```python
from build123d import *

# Parameters (mm, degrees)
F0_W         = 16
F0_H         = 7.6
F1_DEPTH     = 3
F2_R         = 1.1
F3_DEPTH     = 1.7
F5_R         = 1.2
F6_DEPTH     = 3
F6_TAPER     = 7
F7_S5_R      = 1.1
F7_T6_DEPTH  = 3
F7_S11_R     = 1.1
F7_T12_DEPTH = 3
F4_W         = 16
F4_H         = 6
F8_DEPTH     = 7.7
F9_R         = 3
F10_DEPTH    = 5
F11_W        = 1.2
F11_H        = 3.5
F12_DEPTH    = 7.7
F13_R        = 1.5
F14_R        = 0.5
F16_DEPTH    = 4.7
F17_DEPTH    = 7.7
F18_SIZE     = 3
F19_R        = 1


# Not quite as in the source:
# - a fillet or chamfer that OpenCascade refuses, or shapes differently, is made with other operations: its cross-section is extruded or revolved along the edge and cut away or added


with BuildPart() as f1:
    # F0 (on Top) → F1 (new body)
    with BuildSketch(Plane.XY):
        Rectangle(F0_W, F0_H)
    extrude(amount=F1_DEPTH)

    # F2 (on face) → F3 (join)
    with BuildSketch(Plane.XY.offset(3)):
        with Locations((-4.75, 0)):
            Circle(F2_R)
        with Locations((4.75, 0)):
            Circle(F2_R)
    extrude(amount=F3_DEPTH)

    # F5 (on face) → F6 (join)
    with BuildSketch(Plane.XY.offset(4.7)):
        with Locations((-4.75, 0)):
            Circle(F5_R)
        with Locations((4.75, 0)):
            Circle(F5_R)
    extrude(amount=F6_DEPTH, taper=F6_TAPER)

    # F7: fillet of radius 0.1 on 2 edges, made by hand


with BuildPart() as f7_tool2:
    # F7_s3 → F7_t4 (revolve)
    with BuildSketch(Plane.XZ):
        with BuildLine():
            ThreePointArc((-3.6630294386, 4.7), (-3.5881338666, 4.7337379952), (-3.5637748235, 4.8121869343))
            Line((-3.5637748235, 4.8121869343), (-3.55, 4.7))
            Line((-3.55, 4.7), (-3.6630294386, 4.7))
        make_face()
    revolve(axis=Axis((-4.75, 0, 4.7), (0, 0, -1)))

    # F7_s5 → F7_t6 (cut, symmetric)
    with BuildSketch(Plane.XY.offset(4.8)):
        with Locations((-4.75, 0)):
            Circle(F7_S5_R)
    extrude(amount=F7_T6_DEPTH, both=True, mode=Mode.SUBTRACT)


with BuildPart() as f1_1:
    add(f1.part)

    # F7_t1: cut F7_tool2
    add(f7_tool2.part, mode=Mode.SUBTRACT)


with BuildPart() as f7_tool8:
    # F7_s9 → F7_t10 (revolve)
    with BuildSketch(Plane.XZ):
        with BuildLine():
            ThreePointArc((5.8369705614, 4.7), (5.9118661334, 4.7337379952), (5.9362251765, 4.8121869343))
            Line((5.9362251765, 4.8121869343), (5.95, 4.7))
            Line((5.95, 4.7), (5.8369705614, 4.7))
        make_face()
    revolve(axis=Axis((4.75, 0, 4.7), (0, 0, -1)))

    # F7_s11 → F7_t12 (cut, symmetric)
    with BuildSketch(Plane.XY.offset(4.8)):
        with Locations((4.75, 0)):
            Circle(F7_S11_R)
    extrude(amount=F7_T12_DEPTH, both=True, mode=Mode.SUBTRACT)


with BuildPart() as f1_2:
    add(f1_1.part)

    # F7_t7: cut F7_tool8
    add(f7_tool8.part, mode=Mode.SUBTRACT)

    # F4 (on Top) → F8 (join, through all)
    with BuildSketch(Plane.XY):
        with Locations((0, 6.8)):
            Rectangle(F4_W, F4_H)
    extrude(amount=F8_DEPTH)

    # F9 (on face) → F10 (join)
    with BuildSketch(Plane(origin=(0, 9.8, 0), x_dir=(-1, 0, 0), z_dir=(0, 1, 0))):
        with BuildLine():
            ThreePointArc((1.6785410332, 0), (3.5135361347, 1.5488994306), (4.2, 3.85))
            ThreePointArc((4.2, 3.85), (3.5135361347, 6.1511005694), (1.6785410332, 7.7))
            Line((1.6785410332, 7.7), (-1.6785410332, 7.7))
            ThreePointArc((-1.6785410332, 7.7), (-4.2, 3.85), (-1.6785410332, 0))
            Line((-1.6785410332, 0), (1.6785410332, 0))
        make_face()
        with Locations((0, 3.85)):
            Circle(F9_R, mode=Mode.SUBTRACT)
    extrude(amount=F10_DEPTH)

    # F11 (on face) → F12 (cut, through all)
    with BuildSketch(Plane.XY.offset(7.7)):
        with Locations((0, 13.05)):
            Rectangle(F11_W, F11_H)
    extrude(amount=-F12_DEPTH, mode=Mode.SUBTRACT)

    # F13
    f13_edges = [f1_2.edges().sort_by_distance(p)[0] for p in [
        (-8, -3.8, 1.5),
        (8, -3.8, 1.5),
    ]]
    fillet(f13_edges, radius=F13_R)

    # F14
    f14_edges = [f1_2.edges().sort_by_distance(p)[0] for p in [
        (-0.6, 11.3, 7.244694),
        (0.6, 11.3, 7.244694),
        (0.6, 11.3, 0.455306),
        (-0.6, 11.3, 0.455306),
    ]]
    fillet(f14_edges, radius=F14_R)

    # F15 (on face) → F16 (cut, through all)
    with BuildSketch(Plane.XY.offset(7.7)):
        with BuildLine():
            ThreePointArc((3.0310889132, 3.8), (3.380740392, 4.6441333421), (3.5, 5.55))
            ThreePointArc((3.5, 5.55), (-0.9058666579, 8.930740392), (-3.0310889132, 3.8))
            Line((-3.0310889132, 3.8), (0, 3.8))
            Line((0, 3.8), (3.0310889132, 3.8))
        make_face()
        with BuildLine():
            ThreePointArc((1.75, 5.55), (1.2374368671, 4.3125631329), (0, 3.8))
            ThreePointArc((0, 3.8), (-1.2374368671, 6.7874368671), (1.75, 5.55))
        make_face(mode=Mode.SUBTRACT)
        with BuildLine():
            ThreePointArc((1.75, 5.55), (-1.2374368671, 6.7874368671), (0, 3.8))
            ThreePointArc((0, 3.8), (1.2374368671, 4.3125631329), (1.75, 5.55))
        make_face()
    extrude(amount=-F16_DEPTH, mode=Mode.SUBTRACT)

    # F15 (on face) → F17 (cut, through all)
    with BuildSketch(Plane.XY.offset(7.7)):
        with BuildLine():
            ThreePointArc((1.75, 5.55), (-1.2374368671, 6.7874368671), (0, 3.8))
            ThreePointArc((0, 3.8), (1.2374368671, 4.3125631329), (1.75, 5.55))
        make_face()
    extrude(amount=-F17_DEPTH, mode=Mode.SUBTRACT)

    # F18
    f18_edges = [f1_2.edges().sort_by_distance(p)[0] for p in [
        (-8, 9.8, 3.85),
        (8, 9.8, 3.85),
    ]]
    chamfer(f18_edges, length=F18_SIZE)

    # F19
    f19_edges = [f1_2.edges().sort_by_distance(p)[0] for p in [
        (-4.2, 9.8, 3.85),
        (4.2, 9.8, 3.85),
    ]]
    fillet(f19_edges, radius=F19_R)


solid = f1_2.part
```
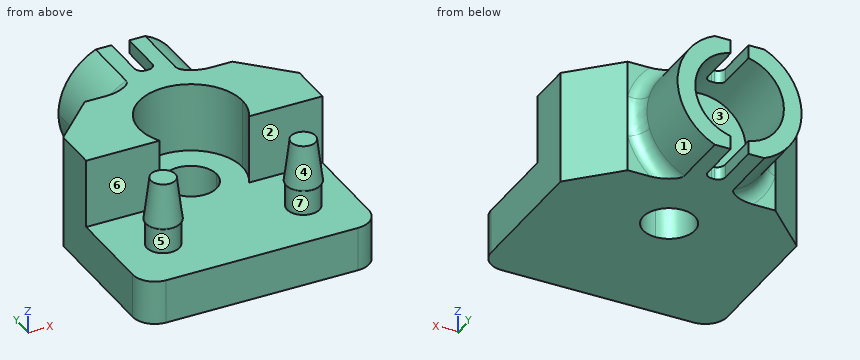
Input: part model. Units: mm. Frame: model coordinates. Face numbers are marked on the shaded views. A direction names the side the tool comes from. Give positions to 0.01 mm unless a question says otherwise; leave off trailing zeros. Order: outer loops, then holes, each group sorted by start corner. A loop starts at its lowest first (then second) coordinate and runs counter-clockwise, first axis right, second up. Notation, with made-up numbers: M -1.5,-5.5 L 6.5,-5.5 A4 cw 6.5,-0.5 Z; hole C 81,87.5 d11. An arc over 180 degrees is marked long. One line per question, with ' | ' between items. Start each with the question number.
1. Section query B-B (z = 6.5). Count the separate pieces of the cut face and the enclosed holes in it, and give its area (3 significant figures).
2. Access query for the marked faces 1, 2 and 3. Directions: +Z, -Z, +X, -X, +Y, -Y. A direction counts if a zero-diameter tool reaches every point of the face in a straight line with its end or side. Return the directions, or none.
3. Pull-direction query (Z, two-part tool) for the marked faces 4, 5, 6 and 7; classes: released by +Z, released by -Z, zero draft, split by the parting line, or undercut.
4. Material intervals for probe 1 along X at (y, z) = (5.55, 4); probe 2 along X at (y, z) = (5.55, 1.1); probe 3 along Y at (x, z) = (0, 5.65), sorted ascending. Write a range as [from, to].
5. First-contact query: pin 1 Ø3 at (x, y) = (0, 5.55) entering from -Z; pin 2 Ø1 at (y, z) = (14, 7) entering from -X; pin 3 Ø1.8 at (x, z) = (-0.5, 2.5) entering from +Y; pin 4 Ø4 at (x, y) = (0.5, 5) entering from +Z. Flat tips, straight axial feed; report the tip coordinate or a pass-through.
6. Section query C-C (y = 8.25). Return the cut outline in (x, z).
7. Section query A-A (y = 0). Return the cut outline in (x, z).
Here are the results:
1) separate pieces: 3 | enclosed holes: 0 | area: 81.1 mm²
2) face 1: +X, +Y | face 2: +Z, +X, -X | face 3: +Y
3) face 4: released by +Z | face 5: undercut | face 6: zero draft | face 7: undercut
4) probe 1: [-8, -3.5], [3.5, 8] | probe 2: [-8, -1.75], [1.75, 8] | probe 3: [9.05, 9.8]
5) pin 1: through | pin 2: x = -3.26 | pin 3: y = 9.8 | pin 4: z = 3
6) outline: M -6.55,0 L 6.55,0 L 6.55,7.7 L 2.23,7.7 L 2.23,3 L -2.23,3 L -2.23,7.7 L -6.55,7.7 Z
7) outline: M -8,0 L 8,0 L 8,3 L 5.85,3 L 5.85,4.7 A0.1 ccw 5.94,4.81 L 5.58,7.7 L 3.92,7.7 L 3.56,4.81 A0.1 ccw 3.65,4.7 L 3.65,3 L -3.65,3 L -3.65,4.7 A0.1 ccw -3.56,4.81 L -3.92,7.7 L -5.58,7.7 L -5.94,4.81 A0.1 ccw -5.85,4.7 L -5.85,3 L -8,3 Z
